Build history of the part. All positions in model axes, mm. Give positions to 0.01 mm unless a question says otherwise; leave off trailing zeros. Loops run counter-clockwise (first coordinate to the right, second up) from the corner with the lowest first, then second, coordinate; pieces in that order, holes last. Notation, with made-up numbers: (2, -13.75) -> (41, -13.75) arc R19 cw to (41, 22.25) -> close; hole circle Ø10 at (-17.5, 14.5). An arc over 180 degrees is marked (long way). One line per question, with ' | ' between items. Start each with the question number.
(1) Slice it at A-A, the plane x = 32.95. Write the cut outline in (y, z) (3 decimals), then the cut area to 3 significant figures.
(2) Slice it at D-D, the plane x = 16.95. Write the cut outline in (y, z) (1 decimal).
(3) Slice it at B-B, the plane y = 32.75. Write the cut outline in (x, z) (3 decimals), then the cut area to 3 significant figures.
(4) Slice it at C-C, the plane z = 0.9. Write the cut outline in (x, y) (3 decimals), then the cut area to 3 significant figures.
(5) Drill centre lines: L1, parallel to Y at x = 32.95, z = 1.25 (3 decimals); L2, parallel to Y at x = 16.95, z = 1.5 (1 decimal); L3, parallel to X at y = 29.5, z = 1.3. Where is each one in solid material? Low to high. Write a range as from..to.
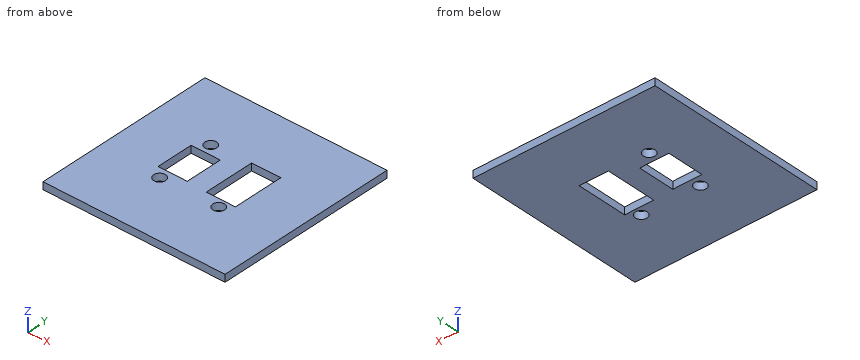
```python
from build123d import *

# Parameters (mm, degrees)
SKETCH1_W           = 50
SKETCH1_H           = 50
BOSS_EXTRUDE1_DEPTH = 2
CUT_EXTRUDE1_REACH  = 72.739
SKETCH2_R           = 1.625
CUT_EXTRUDE2_REACH  = 72.739
SKETCH3_W           = 8
SKETCH3_H           = 10.2
SKETCH3_H_2         = 14


with BuildPart() as part:
    # Sketch1 → Boss-Extrude1 (new body)
    with BuildSketch(Plane.XY):
        with Locations((25, 25)):
            Rectangle(SKETCH1_W, SKETCH1_H)
    extrude(amount=BOSS_EXTRUDE1_DEPTH)

    # Sketch2 → Cut-Extrude1 (cut, up to next)
    with BuildSketch(Plane.XY.offset(2), mode=Mode.PRIVATE) as cut_extrude1_sk1:
        with Locations((16.95, 32.75)):
            Circle(SKETCH2_R)
    cut_extrude1_tool1 = extrude(cut_extrude1_sk1.sketch, amount=-CUT_EXTRUDE1_REACH, mode=Mode.PRIVATE) & part.part
    # Sketch2 → Cut-Extrude1 (cut, up to next)
    with BuildSketch(Plane.XY.offset(2), mode=Mode.PRIVATE) as cut_extrude1_sk2:
        with Locations((16.91, 17)):
            Circle(SKETCH2_R)
    cut_extrude1_tool2 = extrude(cut_extrude1_sk2.sketch, amount=-CUT_EXTRUDE1_REACH, mode=Mode.PRIVATE) & part.part
    # Sketch2 → Cut-Extrude1 (cut, up to next)
    with BuildSketch(Plane.XY.offset(2), mode=Mode.PRIVATE) as cut_extrude1_sk3:
        with Locations((32.95, 17.2)):
            Circle(SKETCH2_R)
    cut_extrude1_tool3 = extrude(cut_extrude1_sk3.sketch, amount=-CUT_EXTRUDE1_REACH, mode=Mode.PRIVATE) & part.part
    add(cut_extrude1_tool1.solids().sort_by_distance((16.95, 32.75, 2))[0], mode=Mode.SUBTRACT)
    add(cut_extrude1_tool2.solids().sort_by_distance((16.91, 17, 2))[0], mode=Mode.SUBTRACT)
    add(cut_extrude1_tool3.solids().sort_by_distance((32.95, 17.2, 2))[0], mode=Mode.SUBTRACT)

    # Sketch3 → Cut-Extrude2 (cut, up to next)
    with BuildSketch(Plane.XY.offset(2), mode=Mode.PRIVATE) as cut_extrude2_sk1:
        with Locations((18, 24.9)):
            Rectangle(SKETCH3_W, SKETCH3_H)
    cut_extrude2_tool1 = extrude(cut_extrude2_sk1.sketch, amount=-CUT_EXTRUDE2_REACH, mode=Mode.PRIVATE) & part.part
    # Sketch3 → Cut-Extrude2 (cut, up to next)
    with BuildSketch(Plane.XY.offset(2), mode=Mode.PRIVATE) as cut_extrude2_sk2:
        with Locations((31.5, 26.5)):
            Rectangle(SKETCH3_W, SKETCH3_H_2)
    cut_extrude2_tool2 = extrude(cut_extrude2_sk2.sketch, amount=-CUT_EXTRUDE2_REACH, mode=Mode.PRIVATE) & part.part
    add(cut_extrude2_tool1.solids().sort_by_distance((18, 24.9, 2))[0], mode=Mode.SUBTRACT)
    add(cut_extrude2_tool2.solids().sort_by_distance((31.5, 26.5, 2))[0], mode=Mode.SUBTRACT)


solid = part.part
```
Final values:
1) outline: (0, 0) -> (15.575, 0) -> (15.575, 2) -> (0, 2) -> close; (18.825, 0) -> (19.5, 0) -> (19.5, 2) -> (18.825, 2) -> close; (33.5, 0) -> (50, 0) -> (50, 2) -> (33.5, 2) -> close | area: 65.5 mm2
2) outline: (0, 0) -> (15.4, 0) -> (15.4, 2) -> (0, 2) -> close; (18.6, 0) -> (19.8, 0) -> (19.8, 2) -> (18.6, 2) -> close; (30, 0) -> (31.1, 0) -> (31.1, 2) -> (30, 2) -> close; (34.4, 0) -> (50, 0) -> (50, 2) -> (34.4, 2) -> close
3) outline: (0, 0) -> (15.325, 0) -> (15.325, 2) -> (0, 2) -> close; (18.575, 0) -> (27.5, 0) -> (27.5, 2) -> (18.575, 2) -> close; (35.5, 0) -> (50, 0) -> (50, 2) -> (35.5, 2) -> close | area: 77.5 mm2
4) outline: (0, 0) -> (50, 0) -> (50, 50) -> (0, 50) -> close; hole (14, 19.8) -> (22, 19.8) -> (22, 30) -> (14, 30) -> close; hole circle Ø3.25 at (16.91, 17); hole circle Ø3.25 at (16.95, 32.75); hole (27.5, 19.5) -> (35.5, 19.5) -> (35.5, 33.5) -> (27.5, 33.5) -> close; hole circle Ø3.25 at (32.95, 17.2) | area: 2,280 mm2
5) L1: 0..15.575, 18.825..19.5, 33.5..50 | L2: 0..15.4, 18.6..19.8, 30..31.1, 34.4..50 | L3: 0..14, 22..27.5, 35.5..50
